Geometry: final body of the model. Coordinates: model frame, mm. Give positions to 0.01 mm unless a question says otherwise; leave off trailing zeros. Loops run counter-clockwise (first coordinate to the right, second up) from the corner with the lowest first, then second, coordinate; pieces in that order, holes last. Notation, with made-up numbers: (45.5, 61.25) - (81.5, 61.25) arc R23 ccw to (81.5, 88.25) - close; hole circle Ø9 at (44, 74). An arc over 180 degrees is marked (long way). Use one line per item in the form item = value.
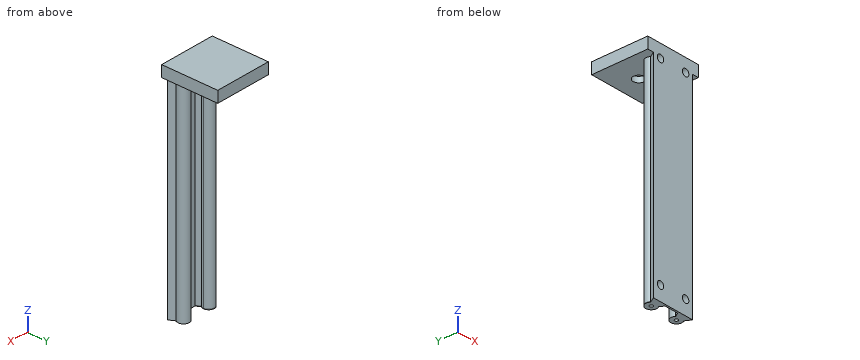
```python
from build123d import *

# Parameters (mm, degrees)
BOSS_EXTRUDE1_DEPTH = 220
BOSS_EXTRUDE4_DEPTH = 220
SKETCH5_R           = 1.37
CUT_EXTRUDE1_DEPTH  = 7
SKETCH6_R           = 1.37
CUT_EXTRUDE2_DEPTH  = 7
CUT_EXTRUDE4_DEPTH  = 10.8
CUT_EXTRUDE5_DEPTH  = 10.8
SKETCH11_R          = 2
CUT_EXTRUDE6_DEPTH  = 7
SKETCH12_R          = 1.5
CUT_EXTRUDE7_DEPTH  = 7
SKETCH13_W          = 50
SKETCH13_H          = 50
BOSS_EXTRUDE5_DEPTH = 10
SKETCH14_R          = 5
CUT_EXTRUDE8_DEPTH  = 5
SKETCH4_2_R         = 3.2
CUT_EXTRUDE9_DEPTH  = 5
SKETCH16_R          = 1.5
BOSS_EXTRUDE7_DEPTH = 0.5


with BuildPart() as part:
    # Sketch1 → Boss-Extrude1 (new body)
    with BuildSketch(Plane.XY):
        with BuildLine():
            ThreePointArc((5, 0), (-1.581139, 4.743416), (-4, -3))
            Line((-4, -3), (4, -3))
            ThreePointArc((4, -3), (4.743416, -1.581139), (5, 0))
        make_face()
        with BuildLine():
            Line((4, -3), (-4, -3))
            ThreePointArc((-4, -3), (0, -5), (4, -3))
        make_face()
        with BuildLine():
            ThreePointArc((5, 0), (-1.581139, 4.743416), (-4, -3))
            Line((-4, -3), (4, -3))
            ThreePointArc((4, -3), (4.743416, -1.581139), (5, 0))
        make_face()
        with BuildLine():
            Line((4, -3), (-4, -3))
            ThreePointArc((-4, -3), (0, -5), (4, -3))
        make_face()
        with BuildLine():
            ThreePointArc((4, -3), (0, -5), (-4, -3))
            Line((-4, -3), (-7, -8.196152))
            Line((-7, -8.196152), (7, -8.196152))
            Line((7, -8.196152), (4, -3))
        make_face()
        with BuildLine():
            Line((28.8, -3), (31.8, -8.196152))
            Line((31.8, -8.196152), (17.8, -8.196152))
            Line((17.8, -8.196152), (20.8, -3))
            ThreePointArc((20.8, -3), (24.8, 5), (28.8, -3))
        make_face()
    extrude(amount=BOSS_EXTRUDE1_DEPTH)

    # Sketch3 → Boss-Extrude4 (add)
    with BuildSketch(Plane.XY.offset(220)):
        Polygon((7, -8.196152), (17.8, -8.196152), (18.65, -8.196152), (18.65, -6.723909), (6.15, -6.723909), (6.15, -8.196152), align=None)
    extrude(amount=-BOSS_EXTRUDE4_DEPTH)

    # Sketch5 → Cut-Extrude1 (cut)
    with BuildSketch(Plane(origin=(0, 0, 0), x_dir=(-1, 0, 0), z_dir=(0, 0, -1))):
        Circle(SKETCH5_R)
        with Locations((-24.8, 0)):
            Circle(SKETCH5_R)
    extrude(amount=-CUT_EXTRUDE1_DEPTH, mode=Mode.SUBTRACT)

    # Sketch6 → Cut-Extrude2 (cut)
    with BuildSketch(Plane.XY.offset(220)):
        with Locations(Location((0, 0, 0), (0, 0, 180))):
            Circle(SKETCH6_R)
        with Locations(Location((24.8, 0, 0), (0, 0, 180))):
            Circle(SKETCH6_R)
    extrude(amount=-CUT_EXTRUDE2_DEPTH, mode=Mode.SUBTRACT)

    # Sketch9 → Cut-Extrude4 (cut)
    with BuildSketch(Plane(origin=(0, 0, 0), x_dir=(-1, 0, 0), z_dir=(0, 0, -1))):
        with BuildLine():
            Line((-28.8, -3), (-31.8, -8.196152))
            Line((-31.8, -8.196152), (7, -8.196152))
            Line((7, -8.196152), (4, -3))
            ThreePointArc((4, -3), (0, 5), (-4, -3))
            Line((-4, -3), (-6.15, -6.723909))
            Line((-6.15, -6.723909), (-18.65, -6.723909))
            Line((-18.65, -6.723909), (-20.8, -3))
            ThreePointArc((-20.8, -3), (-24.8, 5), (-28.8, -3))
        make_face()
    extrude(amount=-CUT_EXTRUDE4_DEPTH, mode=Mode.SUBTRACT)

    # Sketch10 → Cut-Extrude5 (cut)
    with BuildSketch(Plane.XY.offset(220)):
        with BuildLine():
            Line((20.8, -3), (18.65, -6.723909))
            Line((18.65, -6.723909), (6.15, -6.723909))
            Line((6.15, -6.723909), (4, -3))
            ThreePointArc((4, -3), (0, 5), (-4, -3))
            Line((-4, -3), (-7, -8.196152))
            Line((-7, -8.196152), (31.8, -8.196152))
            Line((31.8, -8.196152), (28.8, -3))
            ThreePointArc((28.8, -3), (24.8, 5), (20.8, -3))
        make_face()
    extrude(amount=-CUT_EXTRUDE5_DEPTH, mode=Mode.SUBTRACT)

    # Sketch11 → Cut-Extrude6 (cut)
    with BuildSketch(Plane.XY.offset(209.2)):
        Circle(SKETCH11_R)
        with Locations((24.8, 0)):
            Circle(SKETCH11_R)
    extrude(amount=-CUT_EXTRUDE6_DEPTH, mode=Mode.SUBTRACT)

    # Sketch12 → Cut-Extrude7 (cut)
    with BuildSketch(Plane(origin=(0, 0, 10.8), x_dir=(-1, 0, 0), z_dir=(0, 0, -1))):
        Circle(SKETCH12_R)
        with Locations((-24.8, 0)):
            Circle(SKETCH12_R)
    extrude(amount=-CUT_EXTRUDE7_DEPTH, mode=Mode.SUBTRACT)

    # Sketch13 → Boss-Extrude5 (add)
    with BuildSketch(Plane.XY.offset(209.2)):
        with Locations((12.4, 16.803848)):
            Rectangle(SKETCH13_W, SKETCH13_H)
    extrude(amount=-BOSS_EXTRUDE5_DEPTH)

    # Sketch14 → Cut-Extrude8 (cut)
    with BuildSketch(Plane(origin=(0, 0, 199.2), x_dir=(-1, 0, 0), z_dir=(0, 0, -1))):
        with Locations((-12.4, 22.303848)):
            Circle(SKETCH14_R)
    extrude(amount=-CUT_EXTRUDE8_DEPTH, mode=Mode.SUBTRACT)

    # Sketch4_2 → Cut-Extrude9 (cut)
    with BuildSketch(Plane.XZ.offset(8.196152)):
        with Locations(Location((24.8, 197.5, 0), (0, 0, 270))):
            Circle(SKETCH4_2_R)
        with Locations(Location((24.8, 23.2, 0), (0, 0, 270))):
            Circle(SKETCH4_2_R)
        with Locations(Location((0, 23.2, 0), (0, 0, 270))):
            Circle(SKETCH4_2_R)
        with Locations(Location((0, 197.5, 0), (0, 0, 270))):
            Circle(SKETCH4_2_R)
    extrude(amount=-CUT_EXTRUDE9_DEPTH, mode=Mode.SUBTRACT)

    # Sketch16 → Boss-Extrude7 (add)
    with BuildSketch(Plane(origin=(0, 0, 10.8), x_dir=(-1, 0, 0), z_dir=(0, 0, -1))):
        with BuildLine():
            Line((-31.8, -8.196152), (7, -8.196152))
            Line((7, -8.196152), (4, -3))
            ThreePointArc((4, -3), (0, 5), (-4, -3))
            Line((-4, -3), (-6.15, -6.723909))
            Line((-6.15, -6.723909), (-18.65, -6.723909))
            Line((-18.65, -6.723909), (-20.8, -3))
            ThreePointArc((-20.8, -3), (-24.8, 5), (-28.8, -3))
            Line((-28.8, -3), (-31.8, -8.196152))
        make_face()
        Circle(SKETCH16_R, mode=Mode.SUBTRACT)
        with Locations((-24.8, 0)):
            Circle(SKETCH16_R, mode=Mode.SUBTRACT)
    extrude(amount=BOSS_EXTRUDE7_DEPTH)


solid = part.part
```
(1) Cut plane C-C (y = 32.5). Return the cut outline in (x, z), plus the area to 3 significant figures.
Solution:
outline = (-12.6, 199.2) - (37.4, 199.2) - (37.4, 209.2) - (-12.6, 209.2) - close
area = 500 mm2
(2) Cut plane B-B (z = 23.2). Return the cut outline in (x, y), plus the area to 3 significant figures.
Solution:
outline = (-7, -8.2) - (-3.2, -8.2) - (-3.2, -3.2) - (3.2, -3.2) - (3.2, -8.2) - (21.6, -8.2) - (21.6, -3.2) - (28, -3.2) - (28, -8.2) - (31.8, -8.2) - (28.8, -3) arc R5 ccw (long way) to (20.8, -3) - (18.65, -6.72) - (6.15, -6.72) - (4, -3) arc R5 ccw to (5, 0) arc R5 ccw (long way) to (-4, -3) - close
area = 202 mm2
(3) Pin query (flat end, axial travel): P1, Ø1.5, axis at x = 24.5, y = 0.5, coming from the -Z side; P2, Ø6, axis at x = 0, z = 197.5, coming from the +Y side; P3, Ø7.5, axis at x = 0, z = 23.2, coming from the +Y side; P4, Ø3, axis at x = 1, z = 23.5, coming from the -Y side. Return the tip coordinate at first contact, or that it passes through.
Solution:
P1 = 17.8
P2 = 41.8
P3 = 5
P4 = -3.2
(4) Cut plane D-D (z = 121.5). Return the cut outline in (x, y).
Solution:
outline = (-7, -8.2) - (31.8, -8.2) - (28.8, -3) arc R5 ccw (long way) to (20.8, -3) - (18.65, -6.72) - (6.15, -6.72) - (4, -3) arc R5 ccw to (5, 0) arc R5 ccw (long way) to (-4, -3) - close
(5) Material intervals for L1, parallel to Y at x = 15.5, z = 43.5; L2, parallel to Z at x = -7, y = 23; L3, parallel to Z at x = 13, y = 17.5, sorted ascending. Write a range as from..to.
Solution:
L1 = -8.2..-6.72
L2 = 199.2..209.2
L3 = 204.2..209.2
(6) Cut plane A-A (x = 12.4). Return the cut outline in (y, z).
Solution:
outline = (-8.2, 10.3) - (-6.72, 10.3) - (-6.72, 199.2) - (17.3, 199.2) - (17.3, 204.2) - (27.3, 204.2) - (27.3, 199.2) - (41.8, 199.2) - (41.8, 209.2) - (-8.2, 209.2) - close
